For this review, take the finished solid that the model builds, in its own axes (mm). A direction names the side the tool comes from. Round coordinates to 2 decimals unless told otherwise and drop trailing zeros. Order: outer loops, then holes, each group sorted by start corner. A loop starts at its lowest first (then second) coordinate and runs counter-clockwise, first axis right, second up. Notation, with made-up numbers: M 28.5,55 L 40.5,55 A13 cw 40.5,72 Z; hole C -35.75,30.25 d7. An arc over 180 degrees is marked long. Use a Markdown table: item, result.
from build123d import *

# Parameters (mm, degrees)
SKETCH1_R                       = 15
BOSS_EXTRUDE1_DEPTH             = 6
CUT_EXTRUDE1_REACH              = 24.045
SKETCH2_R                       = 6.125
CBORE_FOR_M3_SHCS2_D            = 3.2
CBORE_FOR_M3_SHCS2_CBORE_D      = 6.5
CBORE_FOR_M3_SHCS2_CBORE_DEPTH  = 3
CIRPATTERN1_COUNT               = 4
BOSS_EXTRUDE2_REACH             = 24.045
BOSS_EXTRUDE2_DIRECTION_2_DEPTH = 20
CUT_EXTRUDE2_START              = -25
SKETCH7_W                       = 15
SKETCH7_H                       = 20
CUT_EXTRUDE2_DEPTH              = 15
BOSS_EXTRUDE3_DEPTH             = 15
CUT_EXTRUDE3_REACH              = 51.759
SKETCH8_R                       = 3


with BuildPart() as part:
    # Sketch1 → Boss-Extrude1 (new body)
    with BuildSketch(Plane(origin=(0, 0, 0), x_dir=(1, 0, 0), z_dir=(0, 1, 0))):
        with Locations(Location((0, 0, 0), (0, 0, 270))):
            Circle(SKETCH1_R)
    extrude(amount=BOSS_EXTRUDE1_DEPTH)

    # Sketch2 → Cut-Extrude1 (cut, up to next)
    with BuildSketch(Plane(origin=(0, 6, 0), x_dir=(1, 0, 0), z_dir=(0, 1, 0)), mode=Mode.PRIVATE) as cut_extrude1_sk1:
        with Locations(Location((0, 0, 0), (0, 0, 270))):
            Circle(SKETCH2_R)
    cut_extrude1_tool1 = extrude(cut_extrude1_sk1.sketch, amount=-CUT_EXTRUDE1_REACH, mode=Mode.PRIVATE) & part.part
    add(cut_extrude1_tool1.solids().sort_by_distance((0, 6, 0))[0], mode=Mode.SUBTRACT)

    # CBORE for M3 SHCS2 (through all)
    with Locations(Plane(origin=(0, 6, 0), x_dir=(1, 0, 0), z_dir=(0, 1, 0))):
        with Locations((0, 9.017)):
            cbore_for_m3_shcs2 = CounterBoreHole(CBORE_FOR_M3_SHCS2_D / 2, CBORE_FOR_M3_SHCS2_CBORE_D / 2, CBORE_FOR_M3_SHCS2_CBORE_DEPTH)

    # CirPattern1: CBORE for M3 SHCS2 ×4 about axis
    cirpattern1_axis = Axis((0, 0, 0), (0, 1, 0))
    for i in range(1, CIRPATTERN1_COUNT):
        add(cbore_for_m3_shcs2.rotate(cirpattern1_axis, i * 360 / CIRPATTERN1_COUNT), mode=Mode.SUBTRACT)

    # Boss-Extrude2: up to this face of the body (flat: up to its plane)
    boss_extrude2_end = Plane(part.part.faces().sort_by_distance((0, 0, -14.575735931))[0])
    # Sketch6 → Boss-Extrude2 (add, up to the picked face)
    with BuildSketch(Plane(origin=(0, 6, 0), x_dir=(1, 0, 0), z_dir=(0, 1, 0)), mode=Mode.PRIVATE) as boss_extrude2_sk1:
        with BuildLine():
            Line((-25, 0), (-25, 15))
            Line((-25, 15), (0, 15))
            ThreePointArc((0, 15), (-10.606601718, 10.606601718), (-15, 0))
            Line((-15, 0), (-25, 0))
        make_face()
    boss_extrude2_tool1 = split(extrude(boss_extrude2_sk1.sketch, amount=-BOSS_EXTRUDE2_REACH, mode=Mode.PRIVATE), bisect_by=boss_extrude2_end, keep=Keep.BOTH, mode=Mode.PRIVATE)
    add(boss_extrude2_tool1.solids().sort_by(Axis((-17.966526, 6, -8.51046), (0, -1, 0)))[0])

    # Sketch6 → Boss-Extrude2 direction 2 (add)
    with BuildSketch(Plane(origin=(0, 6, 0), x_dir=(1, 0, 0), z_dir=(0, 1, 0))):
        with BuildLine():
            Line((-25, 0), (-25, 15))
            Line((-25, 15), (0, 15))
            ThreePointArc((0, 15), (-10.606601718, 10.606601718), (-15, 0))
            Line((-15, 0), (-25, 0))
        make_face()
    extrude(amount=BOSS_EXTRUDE2_DIRECTION_2_DEPTH)

    # Sketch7 → Cut-Extrude2 (cut)
    with BuildSketch(Plane.ZY.offset(25).offset(CUT_EXTRUDE2_START)):
        with Locations((-7.5, 16)):
            Rectangle(SKETCH7_W, SKETCH7_H)
    extrude(amount=CUT_EXTRUDE2_DEPTH, mode=Mode.SUBTRACT)

    # Sketch9 → Boss-Extrude3 (add)
    with BuildSketch(Plane(origin=(0, 0, -15), x_dir=(-1, 0, 0), z_dir=(0, 0, -1))):
        Polygon((15, 26), (15, 6), (0, 6), (0, 0), (25, 0), (25, 26), align=None)
    extrude(amount=BOSS_EXTRUDE3_DEPTH)

    # Sketch8 → Cut-Extrude3 (cut, up to next)
    with BuildSketch(Plane(origin=(-15, 0, 0), x_dir=(0, 0, -1), z_dir=(1, 0, 0)), mode=Mode.PRIVATE) as cut_extrude3_sk1:
        with Locations((18, 18.5)):
            Circle(SKETCH8_R)
    cut_extrude3_tool1 = extrude(cut_extrude3_sk1.sketch, amount=-CUT_EXTRUDE3_REACH, mode=Mode.PRIVATE) & part.part
    add(cut_extrude3_tool1.solids().sort_by_distance((-15, 18.5, -18))[0], mode=Mode.SUBTRACT)


solid = part.part
Q1. Add section C-C (x = 4.5). Write out the cut boundary in (y, z), then the cut area to 3 significant figures.
Determined:
| item | result |
|---|---|
| outline | M 0,-14.31 L 6,-14.31 L 6,-4.16 L 0,-4.16 Z; M 0,4.16 L 6,4.16 L 6,14.31 L 0,14.31 Z |
| area | 122 mm^2 |
Q2. Add section B-B (y = 18.5). Write out the cut boundary in (x, z).
Determined:
| item | result |
|---|---|
| outline | M -25,-30 L -15,-30 L -15,-21 L -25,-21 Z; M -25,-15 L -15,-15 L -15,0 L -25,0 Z |
Q3. Add section A-A (z = -18). Write out the cut boundary in (x, y), then the cut area to 3 significant figures.
Determined:
| item | result |
|---|---|
| outline | M -25,0 L 0,0 L 0,6 L -15,6 L -15,15.5 L -25,15.5 Z; M -25,21.5 L -15,21.5 L -15,26 L -25,26 Z |
| area | 290 mm^2 |
Q4. Clearance check with flat-ended pins moving along their axes: pin 1 (8 mm diameter, centred on y = 18.5, z = -18, fed in from -X); pin 2 (3 mm diameter, centred on x = 9, z = 0.5, fed in from +Y); pin 3 (7.5 mm diameter, centred on x = 0, z = 9.017, fed in from +Y); pin 4 (1.8 mm diameter, centred on y = 3, z = -19, fed in from +X). State where each tip first meets the part, or that it passes through.
Determined:
| item | result |
|---|---|
| pin 1 | stops at x = -25 |
| pin 2 | stops at y = 3 |
| pin 3 | stops at y = 6 |
| pin 4 | stops at x = 0 |
Q5. Wall thickness on line 1 along Y through (x, z) = (-12.5, -2); line 2 along X through (y, z) = (3.5, -28); line 3 along X through (y, z) = (24, -21.5): over which ranges is each line inside the solid? List them lowest first. Write a range as [from, to].
Determined:
| item | result |
|---|---|
| line 1 | y = [0, 6] |
| line 2 | x = [-25, 0] |
| line 3 | x = [-25, -15] |
Q6. Add section D-D (z = -11.5). Write out the cut boundary in (x, y).
Determined:
| item | result |
|---|---|
| outline | M -25,0 L 9.63,0 L 9.63,6 L 2.1,6 L 2.1,3 L -2.1,3 L -2.1,6 L -15,6 L -15,26 L -25,26 Z |
Q7. Machinability: for faces 1 (the flat face through (-1, 3, 11)), 2 (the flat face through (-4, 6, -7)), 3 (the flat face through (-25, 13, -15)), which of the approach directions +Z, -Z, +X, -X, +Y, -Y give a long, thin tool a straight path to every point of the face, cutting with its end or side? Answer none if there is none.
Determined:
| item | result |
|---|---|
| face 1 | +Y |
| face 2 | +Z, -Z, +X, +Y |
| face 3 | +Z, -Z, -X, +Y, -Y |
Q8. Draft analysis for pull direction X (two halves, no side actions). For faces 4 (the cylindrical face through (-0.347, 1.479, 7.455)), 5 (the flat face through (-11, 3, -1)), 6 (the flat face through (0, 3, -22)), 7 (the flat face through (-20, 13, 0)), state which applies: pulls with the +X half, pulls with the -X half, needs draft (parallel to the pull), parting line crosses it, or undercut.
Determined:
| item | result |
|---|---|
| face 4 | undercut |
| face 5 | undercut |
| face 6 | pulls with the +X half |
| face 7 | needs draft |
